Autodesk Inventor part; units mm, degrees
ref_plane "YZ Plane" through (0, 0, 0) normal (1, 0, 0) x (0, 1, 0)
ref_plane "XZ Plane" through (0, 0, 0) normal (0, 1, 0) x (-1, 0, 0)
ref_plane "XY Plane" through (0, 0, 0) normal (0, 0, 1) x (1, 0, 0)
sketch "Sketch1" plane through (0, 0, 0) normal (0, 1, 0) x (-1, 0, 0)
  line L0 (31.678, 204.1316) -> (31.678, 201.3316)
  line L1 (31.678, 201.3316) -> (31.678, 206.9316)
  circle A0 centre (28.8694, 204.1316) radius 2.1
  line L2 (26.7694, 204.1316) -> (30.3694, 204.1316)
  line L3 (30.3694, 204.1316) -> (30.3694, 202.6619)
  line L4 (30.3694, 202.6619) -> (30.3694, 205.6012)
  line L5 (30.3694, 204.1316) -> (31.678, 204.1316)
  line L6 (31.678, 201.3316) -> (34.178, 201.3316)
  line L7 (34.178, 201.3316) -> (34.178, 206.9316)
  line L8 (34.178, 206.9316) -> (31.678, 206.9316)
  line L9 (31.678, 206.9316) -> (31.678, 201.3316)
  circle A1 centre (28.8694, 204.1316) radius 8.5
  circle A2 centre (28.8694, 212.6316) radius 1.55
  circle A3 centre (28.8694, 195.6316) radius 1.55
  line L10 (22.8334, 207.9209) -> (34.9053, 207.9209)
  line L11 (34.9053, 207.9209) -> (34.9053, 200.3422)
  line L12 (34.9053, 200.3422) -> (22.8334, 200.3422)
  line L13 (22.8334, 200.3422) -> (22.8334, 207.9209)
  line L14 (22.8334, 207.9209) -> (34.9053, 200.3422) construction
  line L15 (34.9053, 207.9209) -> (22.8334, 200.3422) construction
  line L16 (22.8334, 200.3422) -> (25.8027, 200.3422)
  line L17 (25.8027, 200.3422) -> (25.8027, 207.9209)
  line L18 (25.8027, 207.9209) -> (22.8334, 207.9209)
  line L19 (22.8334, 207.9209) -> (22.8334, 200.3422)
  dimension "d1" = 2.8
  dimension "d2" = 5.6
  dimension "d3" = 4.2
  dimension "d5" = 2.5
  dimension "d6" = 17
  dimension "d7" = 3.1
  dimension "d8" = 3.1
extrude "Extrusion1" add sketch "Sketch1" along normal blind 7 contours L10 L11 L12 L17
sketch "Sketch2" plane through (0, 0, 0) normal (0, -1, 0) x (1, 0, 0)
  point P0 (0, 0)
sketch "Sketch3" plane through (0, 0, 0) normal (0, -1, 0) x (1, 0, 0)
  circle A0 centre (-28.8694, 204.1316) radius 2.1
  circle A1 centre (-28.8694, 204.1316) radius 8.5
  circle A2 centre (-28.8694, 212.6316) radius 1.55
  circle A3 centre (-28.8694, 195.6316) radius 1.55
  circle A4 centre (-28.8694, 212.6316) radius 3
  circle A5 centre (-28.8694, 195.6316) radius 3
  line L0 (-31.8694, 212.6316) -> (-31.8694, 195.6316)
  line L1 (-25.8694, 195.6316) -> (-25.8694, 212.6316)
  point P0 (0, 0)
  point P1 (-25.9164, 212.1021)
  point P2 (-31.8223, 212.1021)
  point P3 (-31.8694, 212.0845)
  point P4 (-31.8694, 196.1786)
  point P5 (-31.8223, 196.161)
  point P6 (-25.9164, 196.161)
  point P7 (-25.8694, 196.1786)
  point P8 (-25.8694, 212.0845)
  dimension "d11" = 17
  dimension "d12" = 3.1
  dimension "d13" = 3.1
  dimension "d14" = 6
  dimension "d15" = 6
extrude "Extrusion4" add sketch "Sketch3" along normal blind 2.3 contours L1 A1 A5 L0 A4 | A1 A4 L1 | L1 A5 A1 | A4 A1 A2 | A1 A2 A4 | A5 A1 A3 | A1 A3 A5 | A1 L0 A4 | A5 L0 A1
sketch "Sketch5" plane through (0, 0, 0) normal (0, -1, 0) x (1, 0, 0)
  line L0 (-34.9053, 207.9209) -> (-25.8027, 207.9209)
  line L1 (-31.8694, 200.3422) -> (-31.8694, 201.3316)
  line L2 (-34.9053, 207.9209) -> (-31.8694, 207.9209)
  line L3 (-31.8694, 207.9209) -> (-31.8694, 200.3422)
  line L4 (-31.8694, 200.3422) -> (-34.9053, 200.3422)
  line L5 (-34.9053, 200.3422) -> (-34.9053, 207.9209)
  line L6 (-34.178, 201.3316) -> (-31.678, 201.3316)
  line L7 (-31.678, 206.9316) -> (-34.178, 206.9316)
  line L8 (-34.178, 201.3316) -> (-31.8694, 201.3316)
  line L9 (-31.8694, 201.3316) -> (-31.8694, 206.9316)
  line L10 (-31.8694, 206.9316) -> (-34.178, 206.9316)
  line L11 (-34.178, 206.9316) -> (-34.178, 201.3316)
  point P0 (0, 0)
extrude "Extrusion5" add sketch "Sketch5" along normal blind 2.3 contours L0 L3 L7 L11 L6 L1 L4 L5
sketch "Sketch6" plane through (-25.8694, 0, 200.3422) normal (1, 0, 0) x (0, 0, -1)
  line L0 (-9.2808, 8.2816) -> (1.9224, 8.2816)
  line L1 (1.9224, 8.2816) -> (1.9224, -4.0318)
  line L2 (1.9224, -4.0318) -> (-9.2808, -4.0318)
  line L3 (-9.2808, -4.0318) -> (-9.2808, 8.2816)
  point P0 (200.3422, 0)
extrude "Extrusion6" cut sketch "Sketch6" along normal blind 2.3
sketch "Sketch7" plane through (-25.8694, 0, 212.6316) normal (1, 0, 0) x (0, 0, -1)
  point P0 (212.6316, 0)
sketch "Sketch8" plane through (0, 7, 0) normal (0, 1, 0) x (1, 0, 0)
  line L0 (-31.678, -201.3316) -> (-31.678, -206.9316)
  line L1 (-31.678, -206.9316) -> (-34.178, -206.9316)
  line L2 (-34.178, -206.9316) -> (-34.178, -201.3316)
  line L3 (-34.178, -201.3316) -> (-31.678, -201.3316)
  circle A0 centre (-28.8694, -204.1316) radius 2.1
  line L4 (-25.8694, -207.9209) -> (-25.8694, -200.3422)
  line L5 (-25.8694, -200.3422) -> (-34.9053, -200.3422)
  line L6 (-34.9053, -200.3422) -> (-34.9053, -207.9209)
  line L7 (-34.9053, -207.9209) -> (-25.8694, -207.9209)
  point P0 (0, 0)
extrude "Extrusion7" cut sketch "Sketch8" against normal blind 1.7
sketch "Sketch9" plane through (0, 5.3, 0) normal (0, 1, 0) x (1, 0, 0)
  line L0 (-31.678, -201.3316) -> (-31.678, -206.9316)
  line L1 (-34.178, -206.9316) -> (-31.8694, -206.9316)
  line L2 (-31.678, -201.3316) -> (-34.178, -201.3316)
  line L3 (-34.178, -201.3316) -> (-34.178, -206.9316)
  line L4 (-34.178, -206.9316) -> (-31.678, -206.9316)
  line L5 (-31.678, -206.9316) -> (-31.678, -201.3316)
  point P0 (0, 0)
extrude "Extrusion8" cut sketch "Sketch9" against normal through all
sketch "Sketch10" plane through (-34.9053, -2.3, 200.3422) normal (-1, 0, 0) x (0, 0, 1)
  line L0 (6.5893, 7.6) -> (0.9893, 7.6)
  line L1 (3.7893, 7.6) -> (3.7893, 0)
  line L2 (5.8893, 0) -> (1.6893, 0)
  line L3 (3.7893, 2.0731) -> (3.7893, 5.5269) construction
  line L4 (3.7893, 3.8) -> (3.7893, 2.7114)
  line L5 (3.7893, 4.8886) -> (3.7893, 2.7114) construction
  line L6 (2.1893, 4.8886) -> (2.1893, 2.7114)
  line L7 (5.3893, 2.7114) -> (5.3893, 4.8886)
  arc A0 (5.3893, 4.8886) -> (2.1893, 4.8886) centre (3.7893, 4.8886) ccw
  arc A1 (2.1893, 2.7114) -> (5.3893, 2.7114) centre (3.7893, 2.7114) ccw
  point P0 (-200.3422, 2.3)
  dimension "d39" = 3.2
fillet "Fillet1" radius 0.7 2 edges at (-34.9053, 1.5, 207.9209) (-34.9053, 1.5, 200.3422)
fillet "Fillet2" radius 1 2 edges at (-25.8694, 2.65, 207.9209) (-25.8694, 2.65, 200.3422)
sketch "Sketch11" plane through (0, 5.3, 0) normal (0, 1, 0) x (1, 0, 0)
  circle A0 centre (-28.8694, -204.1316) radius 2.1
  circle A1 centre (-28.8694, -204.1316) radius 2.1
  line L0 (-26.7694, -204.1316) -> (-30.4694, -204.1316)
  line L1 (-30.4694, -204.1316) -> (-30.4694, -202.7714)
  line L2 (-30.4694, -202.7714) -> (-30.4694, -205.4917)
  point P0 (0, 0)
  dimension "d36" = 3.7
extrude "Extrusion10" add sketch "Sketch11" against normal up to surface (7.6 mm away) contours L1 L2 A0
extrude "Extrusion11" cut sketch "Sketch10" against normal blind 6
sketch "Sketch12" plane through (0, 5.3, 0) normal (0, 1, 0) x (1, 0, 0)
  circle A0 centre (-28.8694, -212.6316) radius 1.55
  circle A1 centre (-28.8694, -212.6316) radius 3
  circle A2 centre (-28.8694, -195.6316) radius 1.55
  circle A3 centre (-28.8694, -195.6316) radius 3
  arc A4 (-30.4694, -205.4917) -> (-30.4694, -202.7714) centre (-28.8694, -204.1316) ccw
  circle A5 centre (-28.8694, -204.1316) radius 6.9874
  arc A6 (-25.8694, -201.3422) -> (-26.8694, -200.3422) centre (-26.8694, -201.3422) ccw
  line L0 (-34.2053, -200.3422) -> (-26.8694, -200.3422)
  arc A7 (-34.2053, -200.3422) -> (-34.9053, -201.0422) centre (-34.2053, -201.0422) ccw
  line L1 (-34.9053, -207.2209) -> (-34.9053, -201.0422)
  arc A8 (-34.9053, -207.2209) -> (-34.2053, -207.9209) centre (-34.2053, -207.2209) ccw
  line L2 (-26.8694, -207.9209) -> (-34.2053, -207.9209)
  arc A9 (-26.8694, -207.9209) -> (-25.8694, -206.9209) centre (-26.8694, -206.9209) ccw
  line L3 (-25.8694, -201.3422) -> (-25.8694, -206.9209)
  line L4 (-31.678, -206.9316) -> (-31.678, -201.3316)
  line L5 (-34.178, -206.9316) -> (-31.678, -206.9316)
  line L6 (-34.178, -201.3316) -> (-34.178, -206.9316)
  line L7 (-31.678, -201.3316) -> (-34.178, -201.3316)
  arc A10 (-30.4694, -205.4917) -> (-30.4694, -202.7714) centre (-28.8694, -204.1316) ccw
  line L8 (-30.4694, -205.4917) -> (-30.4694, -202.7714)
  point P0 (0, 0)
  point P1 (-31.1849, -197.539)
  point P2 (-31.1849, -210.7242)
  point P3 (-26.5538, -210.7242)
  point P4 (-26.5538, -197.539)
  dimension "d42" = 6
  dimension "d43" = 6
extrude "Extrusion12" add sketch "Sketch12" against normal up to surface (7.6 mm away) contours A1 A5 A3
sketch "Sketch13" plane through (0, 0, 0) normal (0, 1, 0) x (1, 0, 0)
  circle A0 centre (-28.8694, -212.6316) radius 1.55
  circle A1 centre (-28.8694, -212.6316) radius 4
  circle A2 centre (-28.8694, -195.6316) radius 1.55
  circle A3 centre (-28.8694, -195.6316) radius 4
  line L0 (-32.8694, -212.6316) -> (-32.8694, -195.6316)
  line L1 (-24.8694, -212.6316) -> (-24.8694, -195.6316)
  line L2 (-31.678, -201.3316) -> (-34.178, -201.3316)
  line L3 (-34.178, -206.9316) -> (-31.678, -206.9316)
  line L4 (-31.678, -201.3316) -> (-32.928, -201.3316)
  line L5 (-32.928, -201.3316) -> (-32.928, -206.9316)
  line L6 (-32.928, -206.9316) -> (-31.678, -206.9316)
  line L7 (-31.678, -206.9316) -> (-31.678, -201.3316)
  point P0 (0, 0)
  point P1 (-32.8694, -201.3316)
  point P2 (-32.8694, -206.9316)
  dimension "d46" = 8
  dimension "d47" = 8
extrude "Extrusion13" add sketch "Sketch13" against normal up to surface (2.3 mm away) contours A1 | A1 L0 L3 L7 L2 A3 L1 | A3
sketch "Sketch14" plane through (0, 5.3, 0) normal (0, 1, 0) x (1, 0, 0)
  line L0 (-24.8694, -212.6316) -> (-24.8694, -209.8608)
  line L1 (-24.8694, -198.4023) -> (-24.8694, -195.6316)
  line L2 (-24.8694, -209.8608) -> (-24.8694, -198.4023)
  line L3 (-24.8694, -198.4023) -> (-21.4183, -198.4023)
  line L4 (-21.4183, -198.4023) -> (-21.2342, -210.9453)
  line L5 (-21.2342, -210.9453) -> (-24.8694, -209.8608)
  point P0 (0, 0)
extrude "Extrusion14" cut sketch "Sketch14" against normal through all
sketch "Sketch16" plane through (-34.9053, 0.4114, 202.5316) normal (1, 0, 0) x (0, 0, -1)
  line L0 (0, 0) -> (0, 2.1771)
  arc A0 (0, 2.1771) -> (-3.2, 2.1771) centre (-1.6, 2.1771) ccw
  line L1 (-3.2, 2.1771) -> (-3.2, 0)
  arc A1 (-3.2, 0) -> (0, 0) centre (-1.6, 0) ccw
  point P0 (202.5316, -0.4114)
extrude "Extrusion16" cut sketch "Sketch16" against normal blind 10
sketch "Sketch17" plane through (0, 0, 0) normal (0, 1, 0) x (1, 0, 0)
  arc A0 (-32.8694, -209.8608) -> (-31.1849, -210.7242) centre (-28.8694, -204.1316) ccw
  line L0 (-32.8694, -209.8608) -> (-32.8694, -212.6316)
  arc A1 (-32.8694, -212.6316) -> (-24.8694, -212.6316) centre (-28.8694, -212.6316) ccw
  line L1 (-24.8694, -212.6316) -> (-24.8694, -209.8608)
  arc A2 (-26.5538, -210.7242) -> (-24.8694, -209.8608) centre (-28.8694, -204.1316) ccw
  arc A3 (-26.5538, -210.7242) -> (-31.1849, -210.7242) centre (-28.8694, -212.6316) ccw
  circle A4 centre (-28.8694, -212.6316) radius 1.55
  arc A5 (-31.1849, -197.539) -> (-32.8694, -198.4023) centre (-28.8694, -204.1316) ccw
  arc A6 (-31.1849, -197.539) -> (-26.5538, -197.539) centre (-28.8694, -195.6316) ccw
  arc A7 (-24.8694, -198.4023) -> (-26.5538, -197.539) centre (-28.8694, -204.1316) ccw
  line L2 (-24.8694, -198.4023) -> (-24.8694, -195.6316)
  arc A8 (-24.8694, -195.6316) -> (-32.8694, -195.6316) centre (-28.8694, -195.6316) ccw
  line L3 (-32.8694, -195.6316) -> (-32.8694, -198.4023)
  circle A9 centre (-28.8694, -195.6316) radius 1.55
  point P0 (0, 0)
extrude "Extrusion17" add sketch "Sketch17" along normal blind 1
sketch "Sketch18" plane through (0, 0, 0) normal (0, 1, 0) x (1, 0, 0)
  line L0 (-30.2904, -205.6777) -> (-31.678, -205.6777)
  arc A0 (-30.2904, -205.6777) -> (-30.2904, -202.5854) centre (-28.8694, -204.1316) ccw
  line L1 (-31.678, -202.5854) -> (-30.2904, -202.5854)
  line L2 (-31.678, -202.5854) -> (-31.678, -205.6777)
  point P0 (0, 0)
sketch "Sketch19" plane through (0, 5.3, 0) normal (0, 1, 0) x (1, 0, 0)
  line L0 (-30.4694, -205.4917) -> (-30.4694, -202.7714)
  arc A0 (-30.4694, -205.4917) -> (-30.4694, -202.7714) centre (-28.8694, -204.1316) ccw
  point P0 (0, 0)
extrude "Extrusion18" cut sketch "Sketch19" against normal through all
sketch "Sketch20" plane through (0, 5.3, 0) normal (0, 1, 0) x (1, 0, 0)
  point P0 (0, 0)
properties part number "Acople3"
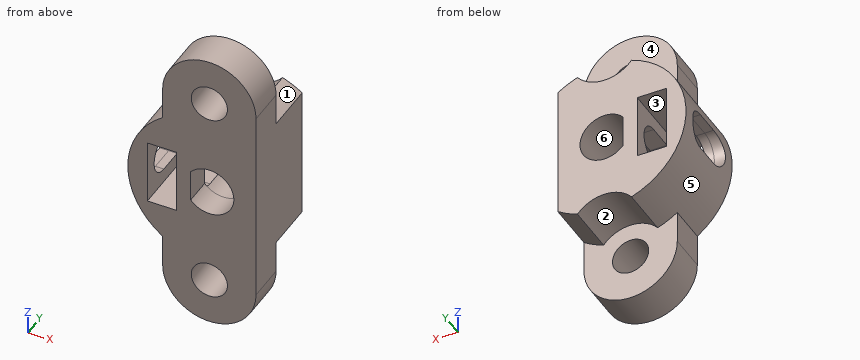
Geometry check sheet. Reference: the model listing, model coordinates, mm. Face numbers are marked on the shaded views. A direction names the side the tool comes from. Coordinates: 2 decimals unless noted, no trailing zeros. Write each loop counter-clockwise with the first axis right and the second up, starting at its lowest first coordinate (ties: lowest second). Pieces come first, ordered by that corner, then holes. Notation, with made-up numbers: M 63.5,32.25 L 94.5,32.25 A21 ccw 94.5,58.25 Z; hole C 40,67.25 d7. An arc over 180 degrees is marked long. Use one line per item in the form item = value. Start each with the question number.
1) Section check C-C on z = 213.75. Enter the section's corners in (x, y).
2) Release check for a two-part mould opening along Z. For the marked faces 4, 5 and 6 record: pulls with the +Z half, pulls with the -Z half, needs draft (parallel to the pull), parting line crosses it, or undercut.
3) Section check D-D on x = -32.5. Enter the section's corners in (y, z).
4) Section check A-A on y = -1.75. Enter the section's corners in (x, z).
5) Thickness scan on probe 1 along X at (y, z) = (0, 206); probe 2 along Y at (x, z) = (-30, 193.75); probe 3 along Z at (x, y) = (-29.75, -1). Record the ranges inside material, lowest first. Write a range as from..to.
6) Set-up check for the marked faces 1, 2 and 3: record each of +Z, -Z, +X, -X, +Y, -Y from which the full face is reachable in a straight line by a thin tool's end or side.
7) Section check B-B on x = -30. Enter the section's corners in (y, z).
8) Go/stop test with flat-tipped pins: pin 1 Ø0.7 at (x, y) = (-33.5, 2.5) entering from +Z; pin 2 Ø4 at (x, z) = (-28.87, 212.63) entering from +Y; pin 3 Ø0.6 at (x, y) = (-35, 2) entering from -Z. Record where each tip stops, or that it passes through.
Responses:
q1.outline = M -32.71,-2.3 L -29.94,-2.3 L -29.94,1 L -32.71,1 Z; M -27.8,-2.3 L -25.03,-2.3 L -25.03,1 L -27.8,1 Z
q2.face_4 = needs draft
q2.face_5 = parting line crosses it
q2.face_6 = undercut
q3.outline = M -2.3,193.95 L 1,193.95 L 1,198.16 L 5.3,198.16 L 5.3,201.33 L -2.3,201.33 Z; M -2.3,206.93 L 5.3,206.93 L 5.3,210.1 L 1,210.1 L 1,214.31 L -2.3,214.31 Z
q4.outline = M -32.87,195.63 A4 ccw -24.87,195.63 L -24.87,212.63 A4 ccw -32.87,212.63 L -32.87,209.86 A6.99 ccw -32.87,198.4 Z; hole M -34.18,201.33 L -31.68,201.33 L -31.68,206.93 L -34.18,206.93 Z; hole M -30.47,202.77 A2.1 ccw long -30.47,205.49 Z; hole C -28.87,195.63 d3.1; hole C -28.87,212.63 d3.1
q5.probe_1 = -35.6..-34.18, -31.68..-29.83, -27.91..-24.87
q5.probe_2 = -2.3..1
q5.probe_3 = 191.73..194.36, 196.91..202.23, 206.04..211.36, 213.91..216.53
q6.face_1 = +Z, +X, +Y
q6.face_2 = -Z, +Y
q6.face_3 = +Y, -Y
q7.outline = M -2.3,191.79 L 1,191.79 L 1,194.57 L -2.3,194.57 Z; M -2.3,196.69 L 1,196.69 L 1,198.41 L 5.3,198.41 L 5.3,202.36 L -2.3,202.36 Z; M -2.3,205.9 L 5.3,205.9 L 5.3,209.85 L 1,209.85 L 1,211.57 L -2.3,211.57 Z; M -2.3,213.69 L 1,213.69 L 1,216.47 L -2.3,216.47 Z
q8.pin_1 = 209.65
q8.pin_2 = 1
q8.pin_3 = 200.28
